The model under review builds one solid part; all positions refer to its coordinate system, in mm. A direction names the side the tool comes from. Coordinates: 2 decimals unless noted, no trailing zeros. Order: outer loops, then holes, each group sorted by start corner. A loop starts at its lowest first (then second) coordinate and runs counter-clockwise, first axis right, second up. Notation, with made-up numbers: (81.5, -11.5) -> (116.5, -11.5) arc R26 ccw to (116.5, 25.5) -> close; hole circle Ø11 at (-17.5, -24.5). An arc over 180 degrees is marked (long way). Use one line per item in the form item = value.
from build123d import *

# Parameters (mm, degrees)
SKETCH_1_R               = 26.5
EXTRUDE_1_DEPTH          = 10
SKETCH_5_R               = 2.5
CUT_EXTRUDE_4_DEPTH      = 11
PATTERN_CIRCULAR_1_COUNT = 4
CHAMFER_1_SIZE           = 1
SKETCH_6_W               = 30
SKETCH_6_H               = 30
SKETCH_8_W               = 21
SKETCH_8_H               = 10
CUT_EXTRUDE_5_DEPTH      = 11
SKETCH_9_R               = 2.5
CUT_EXTRUDE_7_DEPTH      = 6
MIRROR_3_COPY_1_SKETCH_R = 2.5
MIRROR_3_COPY_1_DEPTH    = 6
SKETCH_12_R              = 3.5
CUT_EXTRUDE_8_DEPTH      = 3
SKETCH_13_R              = 1.75
CUT_EXTRUDE_9_DEPTH      = 8
CHAMFER_2_SIZE           = 1


with BuildPart() as part:
    # Эскиз1 → Бобышка-Вытянуть1 (new body)
    with BuildSketch(Plane.XY):
        Circle(SKETCH_1_R)
    extrude(amount=EXTRUDE_1_DEPTH)

    # Эскиз5 → Вырез-Вытянуть4 (cut, through all)
    with BuildSketch(Plane.XY.offset(10)):
        with Locations((-15.202795796, 15.202795796)):
            Circle(SKETCH_5_R)
    cut_extrude_4 = extrude(amount=-CUT_EXTRUDE_4_DEPTH, mode=Mode.SUBTRACT)

    # Круговой массив1: Вырез-Вытянуть4 ×4 about axis
    pattern_circular_1_axis = Axis((0, 0, 0), (0, 0, 1))
    for i in range(1, PATTERN_CIRCULAR_1_COUNT):
        add(cut_extrude_4.rotate(pattern_circular_1_axis, i * 360 / PATTERN_CIRCULAR_1_COUNT), mode=Mode.SUBTRACT)

    # Фаска1
    chamfer_1_edges = [part.edges().sort_by_distance(p)[0] for p in [
        (-26.5, 0, 10),
    ]]
    chamfer(chamfer_1_edges, length=CHAMFER_1_SIZE)

    # Эскиз6 → Вырез-Повернуть1 (revolve, cut)
    with BuildSketch(Plane.XY):
        with Locations((15, 36)):
            Rectangle(SKETCH_6_W, SKETCH_6_H)
    cut_revolve_1 = revolve(axis=Axis((0, 0, 0), (0, 1, 0)), mode=Mode.SUBTRACT)

    # Зеркальное отражение1: Вырез-Повернуть1 across plane
    add(cut_revolve_1.mirror(Plane.ZX), mode=Mode.SUBTRACT)

    # Эскиз8 → Вырез-Вытянуть5 (cut, through all)
    with BuildSketch(Plane.XY.offset(10)):
        Rectangle(SKETCH_8_W, SKETCH_8_H)
    extrude(amount=-CUT_EXTRUDE_5_DEPTH, mode=Mode.SUBTRACT)

    # Эскиз9 → Вырез-Вытянуть7 (cut)
    with BuildSketch(Plane(origin=(0, 0, 0), x_dir=(-1, 0, 0), z_dir=(0, 0, -1))):
        with BuildLine():
            Line((28.463229875, -9.5), (24.738633754, -9.5))
            ThreePointArc((24.738633754, -9.5), (21.243895878, -15.841303227), (16.163229875, -21))
            Line((16.163229875, -21), (8.463229875, -21))
            Line((8.463229875, -21), (8.463229875, -29.5))
            Line((8.463229875, -29.5), (18.463229875, -29.5))
            Line((18.463229875, -29.5), (28.463229875, -29.5))
            Line((28.463229875, -29.5), (28.463229875, -19.5))
            Line((28.463229875, -19.5), (28.463229875, -9.5))
        make_face()
        with BuildLine():
            Line((24.738633754, -9.5), (18.463229875, -9.5))
            ThreePointArc((18.463229875, -9.5), (11.392162063, -12.428932188), (8.463229875, -19.5))
            Line((8.463229875, -19.5), (8.463229875, -21))
            Line((8.463229875, -21), (16.163229875, -21))
            ThreePointArc((16.163229875, -21), (21.243895878, -15.841303227), (24.738633754, -9.5))
        make_face()
        with Locations((15.202795796, -15.202795796)):
            Circle(SKETCH_9_R, mode=Mode.SUBTRACT)
    cut_extrude_7 = extrude(amount=-CUT_EXTRUDE_7_DEPTH, mode=Mode.SUBTRACT)

    # Зеркальное отражение2: Вырез-Вытянуть7 across plane
    add(cut_extrude_7.mirror(Plane.ZX), mode=Mode.SUBTRACT)

    # Зеркальное отражение3: Вырез-Вытянуть7 across plane
    add(cut_extrude_7.mirror(Plane(origin=(0, 0, 0), x_dir=(0, 0, 1), z_dir=(1, 0, 0))), mode=Mode.SUBTRACT)

    # Зеркальное отражение3 copy 1 sketch → Зеркальное отражение3 copy 1 (cut)
    with BuildSketch(Plane(origin=(0, 0, 0), x_dir=(1, 0, 0), z_dir=(0, 0, -1))):
        with BuildLine():
            Line((28.463229875, -9.5), (24.738633754, -9.5))
            ThreePointArc((24.738633754, -9.5), (21.243895878, -15.841303227), (16.163229875, -21))
            Line((16.163229875, -21), (8.463229875, -21))
            Line((8.463229875, -21), (8.463229875, -29.5))
            Line((8.463229875, -29.5), (18.463229875, -29.5))
            Line((18.463229875, -29.5), (28.463229875, -29.5))
            Line((28.463229875, -29.5), (28.463229875, -19.5))
            Line((28.463229875, -19.5), (28.463229875, -9.5))
        make_face()
        with BuildLine():
            Line((24.738633754, -9.5), (18.463229875, -9.5))
            ThreePointArc((18.463229875, -9.5), (11.392162063, -12.428932188), (8.463229875, -19.5))
            Line((8.463229875, -19.5), (8.463229875, -21))
            Line((8.463229875, -21), (16.163229875, -21))
            ThreePointArc((16.163229875, -21), (21.243895878, -15.841303227), (24.738633754, -9.5))
        make_face()
        with Locations((15.202795796, -15.202795796)):
            Circle(MIRROR_3_COPY_1_SKETCH_R, mode=Mode.SUBTRACT)
    extrude(amount=-MIRROR_3_COPY_1_DEPTH, mode=Mode.SUBTRACT)

    # Эскиз12 → Вырез-Вытянуть8 (cut)
    with BuildSketch(Plane.XY.offset(10)):
        with Locations((-20, 0)):
            Circle(SKETCH_12_R)
    cut_extrude_8 = extrude(amount=-CUT_EXTRUDE_8_DEPTH, mode=Mode.SUBTRACT)

    # Эскиз13 → Вырез-Вытянуть9 (cut, through all)
    with BuildSketch(Plane.XY.offset(7)):
        with Locations((-20, 0)):
            Circle(SKETCH_13_R)
    cut_extrude_9 = extrude(amount=-CUT_EXTRUDE_9_DEPTH, mode=Mode.SUBTRACT)

    # Зеркальное отражение4: Вырез-Вытянуть8, Вырез-Вытянуть9 across plane
    add(cut_extrude_8.mirror(Plane(origin=(0, 0, 0), x_dir=(0, 0, 1), z_dir=(1, 0, 0))), mode=Mode.SUBTRACT)
    add(cut_extrude_9.mirror(Plane(origin=(0, 0, 0), x_dir=(0, 0, 1), z_dir=(1, 0, 0))), mode=Mode.SUBTRACT)

    # Фаска2
    chamfer_2_edges = [part.edges().sort_by_distance(p)[0] for p in [
        (0, -21, 10),
        (0, 21, 10),
    ]]
    chamfer(chamfer_2_edges, length=CHAMFER_2_SIZE)


solid = part.part
Item 1: To check wall thickness, follow L1, parallel to Y at x = -6, z = 6.25; L2, parallel to Y at x = 20, z = 3.75; L3, parallel to Y at x = -15.5, z = 8.25. State the ranges of each line that lie inside material, in increasing order. Write a range as from..to.
Results found:
L1 = -21..-5, 5..21
L2 = -9.5..-1.75, 1.75..9.5
L3 = -21..-17.69, -12.72..12.72, 17.69..21
Item 2: We need section C-C (x = 0). Write out the cut boundary in (y, z).
Results found:
outline = (-21, 0) -> (-5, 0) -> (-5, 10) -> (-20, 10) -> (-21, 9) -> close; (5, 0) -> (21, 0) -> (21, 9) -> (20, 10) -> (5, 10) -> close
Item 3: We need section A-A (z = 3). Write out the cut boundary in (x, y).
Results found:
outline = (-24.74, -9.5) -> (-18.46, -9.5) arc R10 cw to (-8.46, -19.5) -> (-8.46, -21) -> (8.46, -21) -> (8.46, -19.5) arc R10 cw to (18.46, -9.5) -> (24.74, -9.5) arc R26.5 ccw to (24.74, 9.5) -> (18.46, 9.5) arc R10 cw to (8.46, 19.5) -> (8.46, 21) -> (-8.46, 21) -> (-8.46, 19.5) arc R10 cw to (-18.46, 9.5) -> (-24.74, 9.5) arc R26.5 ccw to start; hole circle Ø3.5 at (-20, 0); hole (-10.5, -5) -> (10.5, -5) -> (10.5, 5) -> (-10.5, 5) -> close; hole circle Ø3.5 at (20, 0)
Item 4: Clearance check with flat-ended pins moving along their axes: pin 1 (1 mm diameter, centred on y = -0.5, z = 4, fed in from +X); pin 2 (0.8 mm diameter, centred on y = 20, z = 3.5, fed in from +X); pin 3 (4.5 mm diameter, centred on x = -15.2, y = 15.2, fed in from -Z); pin 4 (3 mm diameter, centred on y = 15.5, z = 9, fed in from -X). State where each tip first meets the part, or that it passes through.
Results found:
pin_1 = 26.5
pin_2 = 8.46
pin_3 = through
pin_4 = -22.5
Item 5: We need section B-B (y = 0). Write out the cut boundary in (x, z), plus the area to 3 significant figures.
Results found:
outline = (-26.5, 0) -> (-21.75, 0) -> (-21.75, 7) -> (-23.5, 7) -> (-23.5, 10) -> (-25.5, 10) -> (-26.5, 9) -> close; (-18.25, 0) -> (-10.5, 0) -> (-10.5, 10) -> (-16.5, 10) -> (-16.5, 7) -> (-18.25, 7) -> close; (10.5, 0) -> (18.25, 0) -> (18.25, 7) -> (16.5, 7) -> (16.5, 10) -> (10.5, 10) -> close; (21.75, 0) -> (26.5, 0) -> (26.5, 9) -> (25.5, 10) -> (23.5, 10) -> (23.5, 7) -> (21.75, 7) -> close
area = 228 mm²
Item 6: We need section D-D (x = 9.5). Write out the cut boundary in (y, z).
Results found:
outline = (-21, 6) -> (-15.07, 6) -> (-15.07, 0) -> (-5, 0) -> (-5, 10) -> (-20, 10) -> (-21, 9) -> close; (5, 0) -> (15.07, 0) -> (15.07, 6) -> (21, 6) -> (21, 9) -> (20, 10) -> (5, 10) -> close
Item 7: Tool access review of faces 1 (the face through (-11.47, 12.35, 2.96)), 2 (the face through (22, -9.5, 3)), 3 (the face through (-8.463, -20, 3)): name each direction out of +Z, -Z, +X, -X, +Y, -Y from which nothing blocks a thin tool from reaching the whole face with its end or side.
Results found:
face_1 = -Z, -X, +Y
face_2 = -Z, +X, -Y
face_3 = -Z, -X, -Y
